from build123d import *

# Parameters (mm, degrees)
F0_R     = 3.95
F1_DEPTH = 50
F2_R     = 6.75
F2_R_2   = 3.95
F3_DEPTH = 2
F4_R     = 10
F4_R_2   = 6.75
F5_DEPTH = 100
F6_R     = 1.5
F7_DEPTH = 10


with BuildPart() as f1:
    # F0 (on Top) → F1 (new body)
    with BuildSketch(Plane.XY):
        Circle(F0_R)
    extrude(amount=F1_DEPTH)

    # F2 (on face) → F3 (join)
    with BuildSketch(Plane.XY.offset(50)):
        Circle(F2_R)
        Circle(F2_R_2, mode=Mode.SUBTRACT)
        Circle(F2_R_2)
    extrude(amount=F3_DEPTH)

    # F4 (on face) → F5 (join)
    with BuildSketch(Plane.XY.offset(52)):
        Circle(F4_R)
        Circle(F4_R_2, mode=Mode.SUBTRACT)
        Circle(F4_R_2)
    extrude(amount=F5_DEPTH)

    # F6 (on face) → F7 (cut)
    with BuildSketch(Plane.XY.offset(152)):
        with Locations((0, 6)):
            Circle(F6_R)
        with Locations((0, -6)):
            Circle(F6_R)
    extrude(amount=-F7_DEPTH, mode=Mode.SUBTRACT)


solid = f1.part
Check sheet for the modelled part. Datum: model origin and axes. Units: mm. A direction names the side the tool comes from. Give positions to 0.01 mm unless a question says otherwise; leave off trailing zeros. Loops run counter-clockwise (first coordinate to the right, second up) from the corner with the lowest first, then second, coordinate; pieces in that order, holes last. Notation, with made-up numbers: M 27,40 L 34,40 A12 cw 34,44 Z; hole C 22,17.5 d9. An arc over 180 degrees is marked long. Return JSON: item names as keys, results as strings. Group by question number.
1. Cross-section at D-D on x = -5.5. Record the boundary of the cut face in (y, z), plus the area to 3 significant figures.
2. Cross-section at B-B on y = 0. Record the boundary of the cut face in (x, z), plus the area to 3 significant figures.
3. Cross-section at A-A on x = 0. Record the boundary of the cut face in (y, z), plus the area to 3 significant figures.
4. Go/stop test with flat-tipped pins: pin 1 (4 mm diameter, centred on x = 4, z = 101.5, fed in from -Y); pin 2 (10 mm diameter, centred on x = -6, z = 120.5, fed in from -Y); pin 3 (0.9 mm diameter, centred on x = 0, y = -6.5, fed in from +Z). Record where each tip stops, or that it passes through.
5. Tool access check on faces 1 (the cylindrical face through (-1.46, -6.59, 50.99)), 2 (the cylindrical face through (-0.325, 4.536, 147.07)), 3 (the flat face through (0, 0, 0)). Record the directions out of +Z, -Z, +X, -X, +Y, -Y that give a thin tool (end or side, any length) a straight path to the whole face; none if there is none.
6. Thickness scan on L1, parallel to Y at x = 0, z = 149.25; L2, parallel to Z at x = 0, y = -7; L3, parallel to Z at x = 0.5, y = 5. Record the ranges inside material, lowest first.
7. Mould release check, pull along Y, two halves, no side actions. Record for faces 4 (the flat face through (0, -6, 142)), 5 (the flat face through (3, -3, 50)), 6 (the cylindrical face through (-2.17, -9.76, 101.3)): released by +Y, released by -Y, zero draft, split by the parting line, or undercut.
8. Cross-section at C-C on z = 43. Record the boundary of the cut face in (x, y).
Return value:
{
 "1": {"outline": "M -8.35,52 L -3.91,52 L -3.91,50 L 3.91,50 L 3.91,52 L 8.35,52 L 8.35,152 L -8.35,152 Z", "area": "1,690 mm^2"},
 "2": {"outline": "M -10,52 L -6.75,52 L -6.75,50 L -3.95,50 L -3.95,0 L 3.95,0 L 3.95,50 L 6.75,50 L 6.75,52 L 10,52 L 10,152 L -10,152 Z", "area": "2,420 mm^2"},
 "3": {"outline": "M -10,52 L -6.75,52 L -6.75,50 L -3.95,50 L -3.95,0 L 3.95,0 L 3.95,50 L 6.75,50 L 6.75,52 L 10,52 L 10,152 L 7.5,152 L 7.5,142 L 4.5,142 L 4.5,152 L -4.5,152 L -4.5,142 L -7.5,142 L -7.5,152 L -10,152 Z", "area": "2,360 mm^2"},
 "4": {"pin 1": "y = -9.8", "pin 2": "y = -9.95", "pin 3": "z = 142"},
 "5": {"face 1": "-Z", "face 2": "+Z", "face 3": "-Z, +X, -X, +Y, -Y"},
 "6": {"L1": "-10 to -7.5, -4.5 to 4.5, 7.5 to 10", "L2": "52 to 142", "L3": "50 to 142"},
 "7": {"face 4": "undercut", "face 5": "zero draft", "face 6": "split by the parting line"},
 "8": {"outline": "C 0,0 d7.9"}
}
